from build123d import *

# Parameters (mm, degrees)
PAD005_DEPTH      = 31
PAD005_DEPTH_BACK = 1
SKETCH022_R       = 11.2
POCKET006_DEPTH   = 15.7868758107
SKETCH030_R       = 0.8
POCKET012_DEPTH   = 12


with BuildPart() as part:
    # Sketch017 → Pad005 (new body, two sides)
    with BuildSketch(Plane.XY) as pad005_sk:
        Polygon((-43.4480411338, -67.1734152894), (-9.9773746751, -77.4064249547), (-8.2231444467, -71.6685964189), (-41.6938109054, -61.4355867536), align=None)
    extrude(amount=PAD005_DEPTH)
    extrude(pad005_sk.sketch, amount=-PAD005_DEPTH_BACK)

    # Sketch022 → Pocket006 (cut, through all)
    with BuildSketch(Plane(origin=(-22.4954398558, -73.5792683564, 0), x_dir=(0.956304756, -0.2923717047, 0), z_dir=(-0.2923717047, -0.956304756, 0))):
        with Locations((-4.4099624333, 31)):
            Circle(SKETCH022_R)
    extrude(amount=-POCKET006_DEPTH, mode=Mode.SUBTRACT)

    # Sketch030 → Pocket012 (cut)
    with BuildSketch(Plane.XY.offset(31)):
        with Locations((-12.610661593, -73.443591444)):
            Circle(SKETCH030_R)
        with Locations((-39.0489589627, -65.3605927726)):
            Circle(SKETCH030_R)
    extrude(amount=-POCKET012_DEPTH, mode=Mode.SUBTRACT)


solid = part.part
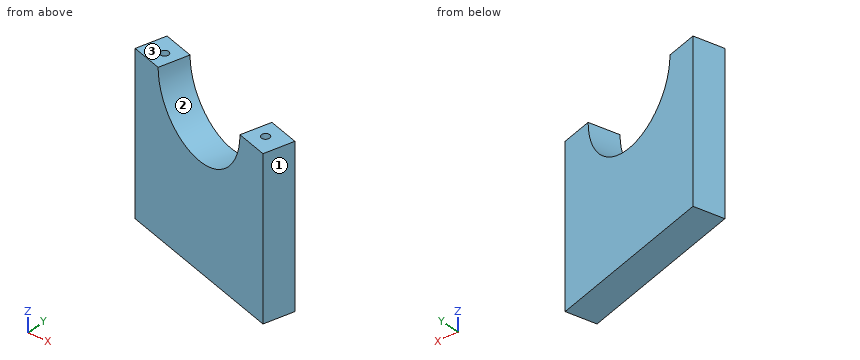
CAD build for the part. Positions are in the model's coordinates, mm. Face numbers are marked on the shaded views. Coordinates: 2 decimals unless noted, no trailing zeros. Write each loop counter-clockwise with the first axis right and the second up, starting at its lowest first coordinate (ties: lowest second). Pieces come first, ordered by that corner, then holes. Notation, with made-up numbers: M 59.25,13.25 L 100.25,13.25 A15 ccw 100.25,34.25 Z; hole C 68,-32.5 d11. An arc over 180 degrees is marked long. Return JSON: item names as keys, results as strings.
Item 1: Slice it at A-A, the plane z = 29. Write the cut outline in (x, y).
Findings below:
{"outline": "M -43.45,-67.17 L -37.25,-69.07 L -35.5,-63.33 L -41.69,-61.44 Z; M -16.17,-75.51 L -9.98,-77.41 L -8.22,-71.67 L -14.42,-69.77 Z; hole C -39.05,-65.36 d1.6; hole C -12.61,-73.44 d1.6"}
Item 2: Two-plate mould, pull along X, no slides. Class the marked faces 1, 2 and 3: +X half, -X half, draft (parallel to the pull), parting line (faces both ways), or undercut.
Findings below:
{"face 1": "+X half", "face 2": "undercut", "face 3": "draft"}
Item 3: Probe line 1 (Z direction, x = -16, y = -70.5); line 2 (Y direction, x = -35.5, z = 10.5); line 3 (Z direction, x = -19.5, y = -72.5). List the from-to ranges inside material, lowest first. Write a range as from..to.
Findings below:
{"line 1": "z = -1..25.44", "line 2": "y = -69.6..-63.33", "line 3": "z = -1..22.22"}
Item 4: Slice it at C-C, the plane z = 18. Write the cut outline in (x, y), and give its area (3 significant figures).
Findings below:
{"outline": "M -43.45,-67.17 L -9.98,-77.41 L -8.22,-71.67 L -41.69,-61.44 Z", "area": "210 mm2"}
Item 5: Drop flat-ended pins along their axis: pin 1 Ø2 at (x, z) = (-29.5, 9.5) entering from +Y; pin 2 Ø8 at (y, z) = (-70, 22) entering from -X; pin 3 Ø5 at (y, z) = (-75, 9.5) entering from +X. Give the stop position or say it passes through.
Findings below:
{"pin 1": "stops at y = -64.86", "pin 2": "stops at x = -43.45", "pin 3": "stops at x = -8.48"}
Item 6: Slice it at D-D, the plane x = -10.5. Write the cut outline in (y, z), and give its area (3 significant figures).
Findings below:
{"outline": "M -77.25,-1 L -70.97,-1 L -70.97,31 L -77.25,31 Z", "area": "201 mm2"}
Item 7: Slice it at B-B, the plane z = 24. Write the cut outline in (x, y).
Findings below:
{"outline": "M -43.45,-67.17 L -35.07,-69.73 L -33.32,-64 L -41.69,-61.44 Z; M -18.35,-74.85 L -9.98,-77.41 L -8.22,-71.67 L -16.6,-69.11 Z; hole C -39.05,-65.36 d1.6; hole C -12.61,-73.44 d1.6"}
